from build123d import *

# Parameters (mm, degrees)
BOSS_EXTRUDE1_DEPTH      = 3.175
BOSS_EXTRUDE1_DEPTH_BACK = 3.175
SKETCH11_R               = 2.5273
SKETCH11_R_2             = 1.7526
CUT_EXTRUDE1_START       = 2.06375
SKETCH12_R               = 2.5273
SKETCH12_R_2             = 2.3749
CUT_EXTRUDE1_DEPTH       = 1.11125
CHAMFER2_SIZE            = 0.3048
CHAMFER2_SIZE2           = 0.527929086
EXTRUDE4_DEPTH           = 5.780702415
EXTRUDE4_DEPTH_BACK      = 5.780702415
SKETCH8_W                = 0.635
SKETCH8_H                = 4.7625


# Read off the part's stored shape, not the designer's step: Cut-Extrude3, Cut-Extrude10
with BuildPart() as part:
    # Sketch11 → Boss-Extrude1 (new, two sides: drawn at the far end of the back side and taken through both)
    with BuildSketch(Plane(origin=(0, 0, 0), x_dir=(1, 0, 0), z_dir=(0, 1, 0)).offset(-BOSS_EXTRUDE1_DEPTH_BACK)):
        with Locations(Location((0, 0, 0), (0, 0, 90))):
            Circle(SKETCH11_R)
        with Locations(Location((0, 0, 0), (0, 0, 90))):
            Circle(SKETCH11_R_2, mode=Mode.SUBTRACT)
    extrude(amount=BOSS_EXTRUDE1_DEPTH + BOSS_EXTRUDE1_DEPTH_BACK)

    # Sketch12 → Cut-Extrude1 (cut)
    with BuildSketch(Plane(origin=(0, 0, 0), x_dir=(1, 0, 0), z_dir=(0, 1, 0)).offset(CUT_EXTRUDE1_START)):
        with Locations(Location((0, 0, 0), (0, 0, 90))):
            Circle(SKETCH12_R)
        with Locations(Location((0, 0, 0), (0, 0, 270))):
            Circle(SKETCH12_R_2, mode=Mode.SUBTRACT)
    extrude(amount=CUT_EXTRUDE1_DEPTH, mode=Mode.SUBTRACT)

    # Cut-Extrude3 outline → Cut-Extrude3 (revolve, cut)
    with BuildSketch(Plane.XY):
        Polygon((1.7526, 3.175), (1.7526, 3.002772478), (1.92786, 3.175), align=None)
    revolve(axis=Axis((0, 0, 0), (0, 1, 0)), mode=Mode.SUBTRACT)

    # Cut-Extrude10 outline → Cut-Extrude10 (revolve, cut)
    with BuildSketch(Plane.XY):
        Polygon((1.92786, -3.175), (1.7526, -3.002772478), (1.7526, -3.175), align=None)
    revolve(axis=Axis((0, 0, 0), (0, 1, 0)), mode=Mode.SUBTRACT)

    # Chamfer2
    chamfer2_edges = [part.edges().sort_by_distance(p)[0] for p in [
        (0, -3.175, 2.5273),
    ]]
    chamfer2_side = [part.faces().sort_by_distance(p)[0] for p in [
        (0, -3.175, 2.455817161),
    ]]
    chamfer(chamfer2_edges, length=CHAMFER2_SIZE, length2=CHAMFER2_SIZE2, reference=chamfer2_side[0])

    # Sketch8 → Extrude4 (cut, two sides: drawn at the far end of the back side and taken through both)
    with BuildSketch(Plane.XY.offset(-EXTRUDE4_DEPTH_BACK)):
        with Locations((0, -0.79375)):
            Rectangle(SKETCH8_W, SKETCH8_H)
    extrude(amount=EXTRUDE4_DEPTH + EXTRUDE4_DEPTH_BACK, mode=Mode.SUBTRACT)


solid = part.part
Build history of the part. All positions in model axes, mm. A direction names the side the tool comes from. Coordinates: 2 decimals unless noted, no trailing zeros. Order: outer loops, then holes, each group sorted by start corner. A loop starts at its lowest first (then second) coordinate and runs counter-clockwise, first axis right, second up. Notation, with made-up numbers: (75, 70.25) - (80, 70.25) arc R6 cw to (80, 77.25) - close; hole circle Ø1 at (40, 52). An arc over 180 degrees is marked (long way). Put each result on its own line as item: value.
1. Pull direction X, two halves, no side cores. Call faces 1 (the face through (2.31, -3.02, 0.05)), 2 (the face through (-0.53, -0.04, -1.67)), 3 (the face through (-0.76, -0.32, -2.41)): pulls with the +X half, pulls with the -X half, needs draft (parallel to the pull), parting line crosses it, or undercut.
Answer sheet:
face 1: pulls with the +X half
face 2: undercut
face 3: parting line crosses it
2. Probe line 1 along X through (y, z) = (-1.75, 0); line 2 along X through (y, z) = (2.5, -0.4); line 3 along Z through (x, y) = (-1.15, 2.75). List the from-to ranges inside material, lowest first. Write a range as [from, to].
Answer sheet:
line 1: x = [-2.53, -1.75], [1.75, 2.53]
line 2: x = [-2.34, -1.71], [1.71, 2.34]
line 3: z = [-2.08, -1.32], [1.32, 2.08]
3. Tool access for faces 4 (the face through (-2.31, -3.02, -0.05)), 5 (the face through (0.713, 2.612, 2.265)): list every direction of +Z, -Z, +X, -X, +Y, -Y with a clear straight run to the whole face (end or side of a thin tool).
Answer sheet:
face 4: -X, -Y
face 5: +Y
4. Drop flat-ended pins along their axis: P1, Ø0.9, axis at y = 0.5, z = 2, coming from the +X side; P2, Ø0.5, axis at x = 0, z = -2, coming from the -Y side; P3, Ø1, axis at x = 1.5, y = -0.5, coming from the +Z side. Give the stop position or say it passes through.
Answer sheet:
P1: stops at x = 2
P2: stops at y = 1.59
P3: stops at z = 2.32
5. Saw through at A-A (y = -1.5). Write the cut outline in (x, z).
Answer sheet:
outline: (-0.32, -2.51) - (-0.32, -1.72) arc R1.75 cw to (-0.32, 1.72) - (-0.32, 2.51) arc R2.53 ccw to start; (0.32, -2.51) arc R2.53 ccw to (0.32, 2.51) - (0.32, 1.72) arc R1.75 cw to (0.32, -1.72) - close
